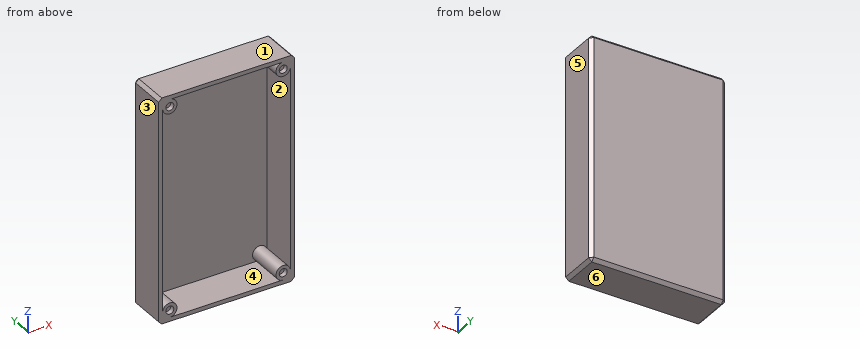
Autodesk Inventor part; units mm, degrees
ref_plane "YZ Plane" through (0, 0, 0) normal (1, 0, 0) x (0, 1, 0)
ref_plane "XZ Plane" through (0, 0, 0) normal (0, 1, 0) x (-1, 0, 0)
ref_plane "XY Plane" through (0, 0, 0) normal (0, 0, 1) x (1, 0, 0)
sketch "Skizze1" plane through (0, 0, 0) normal (0, 1, 0) x (-1, 0, 0)
  line L0 (0, 0) -> (0, -127)
  line L1 (0, -127) -> (71, -127)
  line L2 (71, -127) -> (71, 0)
  line L3 (71, 0) -> (0, 0)
  circle A0 centre (71, 0) radius 2.5
  circle A1 centre (71, -127) radius 2.5
  circle A2 centre (0, -127) radius 2.5
  circle A3 centre (0, 0) radius 2.5
  dimension "d0" = 127
  dimension "d1" = 71
  dimension "d2" = 5
  dimension "d3" = 5
  dimension "d4" = 5
  dimension "d5" = 5
sketch "Skizze2" plane through (0, 0, 0) normal (0, 1, 0) x (-1, 0, 0)
  line L0 (71, -127) -> (71, 0)
  line L1 (71, 0) -> (0, 0)
  line L2 (0, 0) -> (0, -127)
  line L3 (0, -127) -> (71, -127)
  line L4 (78, 7) -> (78, -134)
  line L5 (78, -134) -> (-7, -134)
  line L6 (-7, -134) -> (-7, 7)
  line L7 (-7, 7) -> (78, 7)
  dimension "d6" = 7
extrude "Extrusion1" add sketch "Skizze2" along normal blind 25 contours L3 L2 L1 L0 | L4 L5 L6 L7
extrude "Extrusion2" cut sketch "Skizze1" along normal blind 3 contours L3 A3 L0 | L0 A3 L3 | A2 L1 L0 | L0 L1 A2 | A0 L2 L3 | L3 L2 A0 | A1 L2 L1 | L1 L2 A1
sketch "Skizze3" plane through (0, 0, 0) normal (0, -1, 0) x (1, 0, 0)
  circle A0 centre (-71, -127) radius 2.5
  circle A1 centre (-71, -127) radius 4.5
  circle A2 centre (-71, 0) radius 2.5
  circle A3 centre (-71, 0) radius 4.5
  circle A4 centre (0, 0) radius 2.5
  circle A5 centre (0, 0) radius 4.5
  circle A6 centre (0, -127) radius 2.5
  circle A7 centre (0, -127) radius 4.5
  line L0 (-78, 7) -> (7, 7)
  line L1 (-78, -134) -> (-78, 7)
  line L2 (7, -134) -> (-78, -134)
  line L3 (7, 7) -> (7, -134)
  line L4 (-75.5, 4.5) -> (4.5, 4.5)
  line L5 (4.5, 4.5) -> (4.5, -131.5)
  line L6 (4.5, -131.5) -> (-75.5, -131.5)
  line L7 (-75.5, -131.5) -> (-75.5, 4.5)
  point P0 (-35.5, 7)
  point P1 (-78, -63.5)
  point P2 (-75.5, 0)
  point P3 (-75.5, -127)
  point P4 (-71, -131.5)
  point P5 (0, -131.5)
  point P6 (4.5, -127)
  point P7 (4.5, 0)
  point P8 (0, 4.5)
  point P9 (-71, 4.5)
  dimension "d11" = 9
  dimension "d12" = 9
  dimension "d13" = 9
  dimension "d14" = 9
extrude "Extrusion3" cut sketch "Skizze3" against normal blind 23.5 contours A1 L7 A3 L4 A5 L5 A7 L6
chamfer "Fasen1" distance 2 angle 45 8 edges at (-78, 12.5, -134) (-78, 12.5, 7) (7, 12.5, -134) (7, 12.5, 7) (7, 25, -63.5) (-35.5, 25, 7) (-78, 25, -63.5) (-35.5, 25, -134)
properties part number "LV_Deckel"
Read the model definition and answer for the solid it produces. Units are mm, in the model's axes. Face numbers are marked on the shaded views. A direction names the side the tool comes from. Coordinates: 2 decimals unless noted, no trailing zeros. Loops run counter-clockwise (first coordinate to the right, second up) from the corner with the lowest first, then second, coordinate; pieces in that order, holes last.
Q1. Each of these flat-tipped pins is pushed along its axis until it touches: pin 1 Ø12 at (x, z) = (-67, -19.5) entering from -Y; pin 2 Ø2.5 at (x, z) = (-0.5, -127.5) entering from -Y. Where does it stop, or does it pass through?
Q2. The part is cut by section C-C on x = -51. Write down the section's boundary in (y, z).
Q3. Consider probe 1 along Z at (x, y) = (-24, 11.25); probe 2 along X at (y, z) = (11.25, -116.5); probe 3 along Y at (x, z) = (-74, -71). Determine where each line is inside the solid, lowest interval first.
Q4. The part is cut by section B-B on z = -80. Write down the section's boundary in (x, y).
Q5. The mould has two halves that part along X. Classify the marked faces 3, 4, 5 and 6: +X half, -X half, draft (parallel to the pull), parting line (faces both ways), or undercut.
Q6. The part is cut by section A-A on y = 8.5. Write down the section's boundary in (x, z).
Q7. Which of the six approach directions +Z, -Z, +X, -X, +Y, -Y give full straight-line access (tool end or side, diameter ignored) to the marked faces 1 and 2?
Results below:
1. pin 1: stops at y = 23.5
1. pin 2: stops at y = 3
2. outline: (0, -134) - (23, -134) - (25, -132) - (25, 5) - (23, 7) - (0, 7) - (0, 4.5) - (23.5, 4.5) - (23.5, -131.5) - (0, -131.5) - close
3. probe 1: z = -134 to -131.5, 4.5 to 7
3. probe 2: x = -78 to -75.5, 4.5 to 7
3. probe 3: y = 23.5 to 25
4. outline: (-78, 0) - (-75.5, 0) - (-75.5, 23.5) - (4.5, 23.5) - (4.5, 0) - (7, 0) - (7, 23) - (5, 25) - (-76, 25) - (-78, 23) - close
5. face 3: -X half
5. face 4: undercut
5. face 5: +X half
5. face 6: draft
6. outline: (-78, -132) - (-76, -134) - (5, -134) - (7, -132) - (7, 5) - (5, 7) - (-76, 7) - (-78, 5) - close; hole (-75.5, -127) arc R4.5 cw (long way) to (-71, -131.5) - (0, -131.5) arc R4.5 cw (long way) to (4.5, -127) - (4.5, 0) arc R4.5 cw (long way) to (0, 4.5) - (-71, 4.5) arc R4.5 cw (long way) to (-75.5, 0) - close
7. face 1: +Z, +X, -X, +Y, -Y
7. face 2: -Y
